from build123d import *

# Parameters (mm, degrees)
BOSS_EXTRUDE1_DEPTH   = 3.000000096
SKETCH2_R             = 3.175
CUT_EXTRUDE1_DEPTH    = 4.000000096
SKETCH3_W             = 2.54
SKETCH3_H             = 0.635
CUT_EXTRUDE2_DEPTH    = 4.000000096
BOSS_EXTRUDE2_DEPTH   = 2.206999904
F_6_32_TAPPED_HOLE1_D = 2.7051


with BuildPart() as part:
    # Sketch1 → Boss-Extrude1 (new body)
    with BuildSketch(Plane.XY):
        with BuildLine():
            Line((22.357699804, 50.65759216), (27.218819563, 62.393373411))
            ThreePointArc((27.218819563, 62.393373411), (35.677104191, 57.973626939), (43.43415954, 52.414415661))
            Line((43.43415954, 52.414415661), (67.21146711, 76.191723231))
            ThreePointArc((67.21146711, 76.191723231), (93.866160503, 38.880636728), (101.401368334, -6.35))
            Line((101.401368334, -6.35), (18.648926052, -6.35))
            Line((18.648926052, -6.35), (15.105587123, -4.88230096))
            ThreePointArc((15.105587123, -4.88230096), (14.666587579, 6.075099489), (7.228954972, 14.133571205))
            Line((7.228954972, 14.133571205), (8.696654013, 17.676910134))
            Line((8.696654013, 17.676910134), (34.405475059, 43.38573118))
            ThreePointArc((34.405475059, 43.38573118), (28.61353693, 47.405947816), (22.357699804, 50.65759216))
        make_face()
        with BuildLine():
            Line((88.672924278, 6.35), (27.86051193, 6.35))
            ThreePointArc((27.86051193, 6.35), (26.399857642, 10.93517908), (24.190484974, 15.210228852))
            Line((24.190484974, 15.210228852), (67.191354125, 58.211098004))
            ThreePointArc((67.191354125, 58.211098004), (82.13289044, 34.020557137), (88.672924278, 6.35))
        make_face(mode=Mode.SUBTRACT)
    extrude(amount=BOSS_EXTRUDE1_DEPTH)

    # Sketch2 → Cut-Extrude1 (cut, through all)
    with BuildSketch(Plane.XY.offset(3.000000096)):
        with Locations((22.225, 0)):
            Circle(SKETCH2_R)
        with Locations((36.195, 0)):
            Circle(SKETCH2_R)
        with Locations((61.722, 0)):
            Circle(SKETCH2_R)
        with Locations((75.692, 0)):
            Circle(SKETCH2_R)
        with Locations((95.25, 0)):
            Circle(SKETCH2_R)
        with Locations((15.715448212, 15.715448212)):
            Circle(SKETCH2_R)
        with Locations((25.593729945, 25.593729945)):
            Circle(SKETCH2_R)
        with Locations((43.644044748, 43.644044748)):
            Circle(SKETCH2_R)
        with Locations((53.522326482, 53.522326482)):
            Circle(SKETCH2_R)
        with Locations((92.004434954, 24.652514046)):
            Circle(SKETCH2_R)
        with Locations((82.48891971, 47.625)):
            Circle(SKETCH2_R)
        with Locations((67.351920908, 67.351920908)):
            Circle(SKETCH2_R)
    extrude(amount=-CUT_EXTRUDE1_DEPTH, mode=Mode.SUBTRACT)

    # Sketch3 → Cut-Extrude2 (cut, through all)
    with BuildSketch(Plane.XY.offset(3.000000096)):
        Polygon((15.266435406, 24.246691527), (17.06248663, 26.042742751), (17.511499436, 25.593729945), (15.715448212, 23.797678721), align=None)
        Polygon((44.991083167, 53.971339288), (43.43415954, 52.414415661), (43.883172346, 51.965402855), (45.440095973, 53.522326482), align=None)
        with Locations((29.21, -6.0325)):
            Rectangle(SKETCH3_W, SKETCH3_H)
        with Locations((68.707, -6.0325)):
            Rectangle(SKETCH3_W, SKETCH3_H)
        Polygon((29.230733674, 38.210989795), (31.026784898, 40.007041019), (40.007041019, 31.026784898), (38.210989795, 29.230733674), align=None)
        Polygon((56.845021246, 65.825277367), (55.048970022, 64.029226143), (55.497982828, 63.580213337), (57.294034052, 65.376264561), align=None)
        with Locations((48.9585, -6.0325)):
            Rectangle(SKETCH3_W, SKETCH3_H)
        with Locations((85.471, -6.0325)):
            Rectangle(SKETCH3_W, SKETCH3_H)
        Polygon((99.935462164, 14.437711971), (100.266998693, 11.919442024), (101.526133667, 12.085210288), (101.194597138, 14.603480236), align=None)
        Polygon((93.765504959, 37.464305742), (94.938831965, 37.950313702), (93.966816047, 40.296967714), (92.793489041, 39.810959755), align=None)
        Polygon((79.327792988, 62.471156422), (80.874047017, 60.456038938), (81.88160576, 61.229165953), (80.33535173, 63.244283437), align=None)
        Polygon((13.593916116, 7.005422516), (14.565932035, 4.658768503), (15.739259041, 5.144776462), (14.767243123, 7.491430475), align=None)
    extrude(amount=-CUT_EXTRUDE2_DEPTH, mode=Mode.SUBTRACT)

    # Sketch4 → Boss-Extrude2 (add)
    with BuildSketch(Plane(origin=(0, 0, 0), x_dir=(-1, 0, 0), z_dir=(0, 0, -1))):
        with BuildLine():
            Line((-27.218819563, 62.393373411), (-22.357699804, 50.65759216))
            ThreePointArc((-22.357699804, 50.65759216), (-28.063600293, 47.73355971), (-33.393246405, 44.169553751))
            Line((-33.393246405, 44.169553751), (-42.443492672, 53.219800017))
            ThreePointArc((-42.443492672, 53.219800017), (-35.13186657, 58.305652688), (-27.218819563, 62.393373411))
        make_face()
    extrude(amount=BOSS_EXTRUDE2_DEPTH)

    # #6-32 Tapped Hole1 (through all)
    with Locations(Plane.XY.offset(3.000000096)):
        with Locations((30.861, 53.452819972)):
            Hole(F_6_32_TAPPED_HOLE1_D / 2)


solid = part.part
Can you work these out from the model? Positions are in its coordinate system, mm. A direction names the side the tool comes from. Give positions to 0.01 mm unless a question says otherwise; leave off trailing zeros. Write each loop counter-clockwise with the first axis right and the second up, starting at its lowest first coordinate (ties: lowest second). Pieces come first, ordered by that corner, then holes. Notation, with made-up numbers: M 75,-23 L 107,-23 A9 cw 107,-15 Z; hole C -39,-32 d3. An arc over 180 degrees is marked long. Answer in a Markdown table with one row per item. Add a question column.
Item 1: Imagine slicing it at A-A, the plane y = 0. Write out the boundary of the cut face in (x, z) (3 decimals), plus the area to 3 significant figures.
Item 2: Imagine slicing it at B-B, the plane z = 1.7. State how many separate pieces and enclosed holes the cut face has, plus the area to 3 significant figures.
Item 3: We'd pull the mould along X, two halves only. Please class faces 4 (the flat face through (11.94, 20.92, 1.48)), 5 (the cylindrical face through (25.253, 0.954, 1.521)), 6 (the cylindrical face through (98.094, 26.459, 1.479)): released by +X, released by -X, zero draft, split by the parting line, or undercut.
Item 4: Please list where these lines run through material, in increasing order: L1, parallel to Y at x = 77.5, z = 2.7; L2, parallel to Y at x = 28.5, z = 2.1 (3 decimals); L3, parallel to X at y = 47.5, z = 1.2.
Item 5: On a 3-axis mill with a long thin cutter (end or side, diameter ignored), from which of +Z, -Z, +X, -X, +Y, -Y can I reach the whole of each face in a straight line? I mean faces 1 (the flat face through (35.454, 35.58, 1.521)), 2 (the flat face through (49, -5.715, 2)), 3 (the flat face through (8, 16, 1)). Say none if no direction works.
Item 6: For pin 1 Ø0.5 at (y, z) = (-6, 1.5) entering from +X; pin 2 Ø0.8 at (x, z) = (85, 1) entering from -Y (3 decimals); pin 3 Ø1.5 at (x, z) = (80, -0.5) entering from +Y, each with a flat end and sliding along its axis, tell me the tip position at first contact or that it passes through.
Evaluation:
| question | item | result |
|---|---|---|
| 1 | outline | M 15.875,0 L 19.05,0 L 19.05,3 L 15.875,3 Z; M 25.4,0 L 33.02,0 L 33.02,3 L 25.4,3 Z; M 39.37,0 L 58.547,0 L 58.547,3 L 39.37,3 Z; M 64.897,0 L 72.517,0 L 72.517,3 L 64.897,3 Z; M 78.867,0 L 92.075,0 L 92.075,3 L 78.867,3 Z; M 98.425,0 L 101.6,0 L 101.6,3 L 98.425,3 Z |
| 1 | area | 162 mm² |
| 2 | separate pieces | 1 |
| 2 | enclosed holes | 13 |
| 2 | area | 2,800 mm² |
| 3 | face 4 | released by -X |
| 3 | face 5 | undercut |
| 3 | face 6 | released by +X |
| 4 | L1 | y = -6.35 to -2.61, 2.61 to 6.35, 43.55 to 65.7 |
| 4 | L2 | y = -5.715 to 6.35, 19.52 to 24.315, 26.872 to 37.48, 47.474 to 61.819 |
| 4 | L3 | x = 28.46 to 56.48, 75.15 to 79.32, 85.66 to 89.81 |
| 5 | face 1 | +Z, -Z |
| 5 | face 2 | +Z, -Z, -Y |
| 5 | face 3 | +Z, -Z, -X, +Y |
| 6 | pin 1 | stops at x = 101.44 |
| 6 | pin 2 | stops at y = -5.715 |
| 6 | pin 3 | stops at y = 63.34 |
